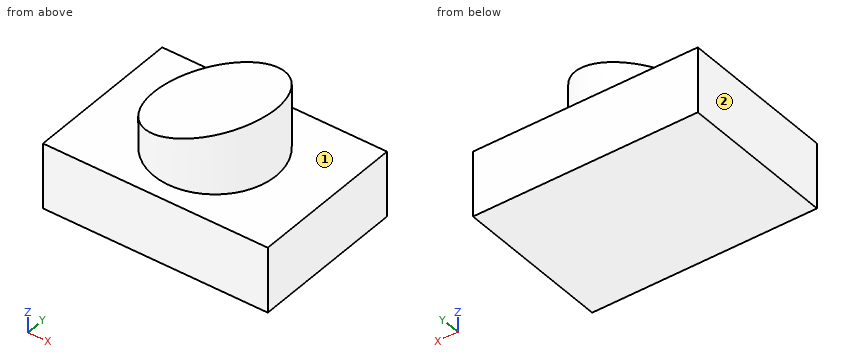
from build123d import *

# Parameters (mm, degrees)
F0_W     = 87.306462
F0_H     = 61.053478
F0_R     = 23.75796
F1_DEPTH = 25.4
F2_R     = 23.75796
F3_DEPTH = 26.162
F5_DEPTH = 61.053477


with BuildPart() as f1:
    # F0 (on Top) → F1 (new body)
    with BuildSketch(Plane.XY):
        Rectangle(F0_W, F0_H)
        Circle(F0_R, mode=Mode.SUBTRACT)
        Circle(F0_R)
    extrude(amount=F1_DEPTH)

    # F2 (on face) → F3 (join)
    with BuildSketch(Plane.XY.offset(25.4)):
        Circle(F2_R)
    extrude(amount=F3_DEPTH)

    # F4 (on face) → F5 (cut, through all)
    with BuildSketch(Plane(origin=(0, 30.526739, 0), x_dir=(-1, 0, 0), z_dir=(0, 1, 0))):
        Polygon((24.116119, 52.158147), (-25.276357, 52.158147), (24.116119, 35.900317), align=None)
    extrude(amount=-F5_DEPTH, mode=Mode.SUBTRACT)


solid = f1.part
The model under review builds one solid part; all positions refer to its coordinate system, in mm. Face numbers are marked on the shaded views. A direction names the side the tool comes from. Round coordinates to 2 decimals unless told otherwise and drop trailing zeros. Write each loop counter-clockwise with the first axis right and the second up, starting at its lowest first coordinate (ties: lowest second). Pieces come first, ordered by that corner, then holes. Notation, with made-up numbers: (2, 88.5) -> (37, 88.5) arc R22 ccw to (37, 126.5) -> close; hole circle Ø7 at (40.25, 83.5). An arc over 180 degrees is marked (long way). Answer as a JSON object with one key per item and string values.
1. We need section B-B on x = -17.5. State the section outline as (y, z) points, and give its area (3 significant figures).
Results found:
{"outline": "(-30.53, 0) -> (30.53, 0) -> (30.53, 25.4) -> (16.07, 25.4) -> (16.07, 38.08) -> (-16.07, 38.08) -> (-16.07, 25.4) -> (-30.53, 25.4) -> close", "area": "1,960 mm^2"}
2. We need section D-D on y = 0. State the section outline as (x, z) points, and give its area (3 significant figures).
Results found:
{"outline": "(-43.65, 0) -> (43.65, 0) -> (43.65, 25.4) -> (23.76, 25.4) -> (23.76, 51.56) -> (23.47, 51.56) -> (-23.76, 36.02) -> (-23.76, 25.4) -> (-43.65, 25.4) -> close", "area": "3,090 mm^2"}
3. To check wall thickness, follow line 1 along Z through (x, y) = (24.5, -7); line 2 along Z through (x, y) = (-6, 19); line 3 along Y through (x, z) = (-3.5, 26.5). State the ranges of each line that lie inside material, in increasing order.
Results found:
{"line 1": "z = 0 to 25.4", "line 2": "z = 0 to 41.86", "line 3": "y = -23.5 to 23.5"}
4. We need section A-A on y = 15.5. State the section outline as (x, z) points.
Results found:
{"outline": "(-43.65, 0) -> (43.65, 0) -> (43.65, 25.4) -> (18.01, 25.4) -> (18.01, 49.76) -> (-18.01, 37.91) -> (-18.01, 25.4) -> (-43.65, 25.4) -> close"}
5. We need section C-C on z = 39.5. State the section outline as (x, y) points, and give its area (3 significant figures).
Results found:
{"outline": "(-13.18, -19.77) arc R23.76 ccw (long way) to (-13.18, 19.77) -> close", "area": "1,480 mm^2"}
6. Machinability: for the marked faces 1 and 2, which of the approach directions +Z, -Z, +X, -X, +Y, -Y give a long, thin tool a straight path to every point of the face, cutting with its end or side? Answer none if there is none.
Results found:
{"face 1": "+Z", "face 2": "+Z, -Z, -X, +Y, -Y"}
7. Clearance check with flat-ended pins moving along their axes: pin 1 (5 mm diameter, centred on x = 12.5, y = -6, fed in from +Z); pin 2 (2 mm diameter, centred on y = -9, z = 28, fed in from +X); pin 3 (10 mm diameter, centred on y = 23, z = 36, fed in from -X). State where each tip first meets the part, or that it passes through.
Results found:
{"pin 1": "stops at z = 48.78", "pin 2": "stops at x = 22.37", "pin 3": "stops at x = -15.51"}
